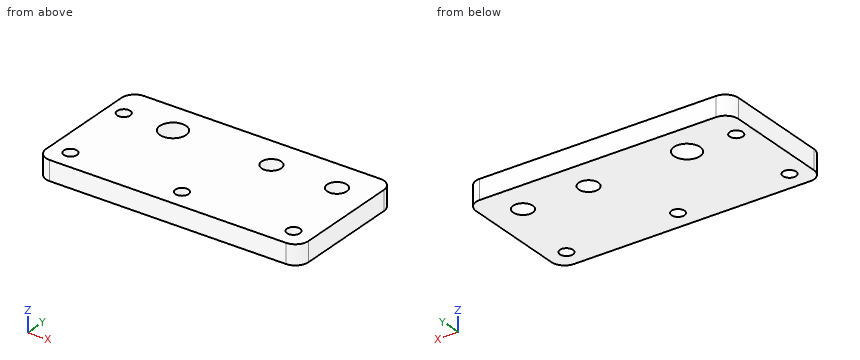
```python
from build123d import *

# Parameters (mm, degrees)
SKETCH_W        = 80
SKETCH_H        = 40
PAD_DEPTH       = 6
SKETCH001_R     = 3
SKETCH001_R_2   = 4
POCKET_DEPTH    = 7
FILLET_R        = 4
FILLET001_R     = 4
FILLET002_R     = 4
FILLET003_R     = 4
SKETCH002_R     = 2
POCKET001_DEPTH = 8


with BuildPart() as part:
    # Sketch → Pad (new body)
    with BuildSketch(Plane.XY):
        with Locations((40, 20)):
            Rectangle(SKETCH_W, SKETCH_H)
    extrude(amount=PAD_DEPTH)

    # Sketch001 → Pocket (cut)
    with BuildSketch(Plane.XY.offset(6)):
        with Locations((50, 30)):
            Circle(SKETCH001_R)
        with Locations((70, 30)):
            Circle(SKETCH001_R)
        with Locations((20, 30)):
            Circle(SKETCH001_R_2)
    extrude(amount=-POCKET_DEPTH, mode=Mode.SUBTRACT)

    # Fillet
    fillet_edges = [part.edges().sort_by_distance(p)[0] for p in [
        (0, 0, 3),
    ]]
    fillet(fillet_edges, radius=FILLET_R)

    # Fillet001
    fillet001_edges = [part.edges().sort_by_distance(p)[0] for p in [
        (80, 0, 3),
    ]]
    fillet(fillet001_edges, radius=FILLET001_R)

    # Fillet002
    fillet002_edges = [part.edges().sort_by_distance(p)[0] for p in [
        (80, 40, 3),
    ]]
    fillet(fillet002_edges, radius=FILLET002_R)

    # Fillet003
    fillet003_edges = [part.edges().sort_by_distance(p)[0] for p in [
        (0, 40, 3),
    ]]
    fillet(fillet003_edges, radius=FILLET003_R)

    # Sketch002 → Pocket001 (cut)
    with BuildSketch(Plane.XY.offset(6)):
        with Locations((5, 30)):
            Circle(SKETCH002_R)
        with Locations((6, 6)):
            Circle(SKETCH002_R)
        with Locations((40, 6)):
            Circle(SKETCH002_R)
        with Locations((74, 6)):
            Circle(SKETCH002_R)
    extrude(amount=-POCKET001_DEPTH, mode=Mode.SUBTRACT)


solid = part.part
```
The model under review builds one solid part; all positions refer to its coordinate system, in mm. Round coordinates to 2 decimals unless told otherwise and drop trailing zeros. Loops run counter-clockwise (first coordinate to the right, second up) from the corner with the lowest first, then second, coordinate; pieces in that order, holes last. Notation, with made-up numbers: M -2.75,62.5 L 27.25,62.5 A22 ccw 27.25,87.5 Z; hole C 27,-15.5 d7. An arc over 180 degrees is marked long. Answer as a JSON object with one key per item and string values.
(1) Take a section at B-B on y = 6. Give the boundary of the cut face in (x, z), and give its area (3 significant figures).
Resolved:
{"outline": "M 0,0 L 4,0 L 4,6 L 0,6 Z; M 8,0 L 38,0 L 38,6 L 8,6 Z; M 42,0 L 72,0 L 72,6 L 42,6 Z; M 76,0 L 80,0 L 80,6 L 76,6 Z", "area": "408 mm²"}
(2) Take a section at A-A on x = 74. Give the boundary of the cut face in (y, z).
Resolved:
{"outline": "M 0,0 L 4,0 L 4,6 L 0,6 Z; M 8,0 L 40,0 L 40,6 L 8,6 Z"}
(3) Take a section at C-C on y = 30. Give the boundary of the cut face in (x, z).
Resolved:
{"outline": "M 0,0 L 3,0 L 3,6 L 0,6 Z; M 7,0 L 16,0 L 16,6 L 7,6 Z; M 24,0 L 47,0 L 47,6 L 24,6 Z; M 53,0 L 67,0 L 67,6 L 53,6 Z; M 73,0 L 80,0 L 80,6 L 73,6 Z"}
(4) To check wall thickness, follow line 1 along Y through (x, z) = (40, 4.2); line 2 along Y through (x, z) = (70, 4.7); line 3 along Y through (x, z) = (5, 2.8). State the ranges of each line that lie inside material, in increasing order.
Resolved:
{"line 1": "0 to 4, 8 to 40", "line 2": "0 to 27, 33 to 40", "line 3": "0 to 4.27, 7.73 to 28, 32 to 40"}
(5) Take a section at D-D on z = 2.9. Give the boundary of the cut face in (x, y).
Resolved:
{"outline": "M 0,4 A4 ccw 4,0 L 76,0 A4 ccw 80,4 L 80,36 A4 ccw 76,40 L 4,40 A4 ccw 0,36 Z; hole C 5,30 d4; hole C 6,6 d4; hole C 20,30 d8; hole C 40,6 d4; hole C 50,30 d6; hole C 70,30 d6; hole C 74,6 d4"}
